```python
from build123d import *

# Parameters (mm, degrees)
F0_R      = 11
F1_DEPTH  = 7
F2_F1_R   = 2.54
F2_F2_R   = 2.54
F7_DEPTH  = 7.001
F8_DEPTH  = 7.001
F9_DEPTH  = 7.001
F10_DEPTH = 7.001


with BuildPart() as f1:
    # F0 (on Top) → F1 (new body)
    with BuildSketch(Plane.XY):
        Polygon((-46.5175881982, -16.4707175266), (1.3742837651, -16.4707175266), (47.8816837651, -16.4707175266), (38.1750466591, -6.3388262363), (28.4684095532, 3.7930650539), (38.1750466591, 13.9249563442), (47.8816837651, 24.0568476345), (1.3742837651, 24.0568476345), (-46.5175881982, 24.0568476345), (-36.8075984385, 13.9249563442), (-27.0976086789, 3.7930650539), (-36.8075984385, -6.3388262363), align=None)
        with Locations((1.3742837651, 3.7930650539)):
            Circle(F0_R, mode=Mode.SUBTRACT)
    extrude(amount=F1_DEPTH)

    # F2: fillet of radius 2.54 on 10 edges, made by hand

    # F2_f1
    f2_f1_edges = [f1.edges().sort_by_distance(p)[0] for p in [
        (28.4684095532, 3.7930650539, 3.5),
        (-27.0976086789, 3.7930650539, 3.5),
    ]]
    fillet(f2_f1_edges, radius=F2_F1_R)

    # F2_f2
    f2_f2_edges = [f1.edges().sort_by_distance(p)[0] for p in [
        (0.6820477835, -16.4707175266, 7),
        (0.6820477835, 24.0568476345, 7),
        (0.6820477835, 24.0568476345, 0),
        (0.6820477835, -16.4707175266, 0),
        (39.0167452033, -7.2174001498, 7),
        (-37.649739308, 14.8036884491, 7),
        (-37.649739308, -7.2175583413, 0),
        (39.0167452033, 14.8035302576, 0),
        (29.4459362755, 3.7930650539, 0),
        (-28.0757168957, 3.7930650539, 0),
        (-28.0757168957, 3.7930650539, 7),
        (29.4459362755, 3.7930650539, 7),
    ]]
    fillet(f2_f2_edges, radius=F2_F2_R)

    # F3 (on face) → F7 (cut, through all)
    with BuildSketch(Plane.XY.offset(7)):
        Polygon((-12.7487120452, 8.4079941735), (-12.7487120452, 16.6059941735), (-19.8483883054, 20.7049941735), (-26.9480645657, 16.6059941735), (-26.9480645657, 8.4079941735), (-19.8483883054, 4.3089941735), align=None)
    extrude(amount=-F7_DEPTH, mode=Mode.SUBTRACT)

    # F4 (on face) → F8 (cut, through all)
    with BuildSketch(Plane.XY.offset(7)):
        Polygon((-12.8069793108, -8.9152967557), (-12.8069793108, -0.7172967557), (-19.906655571, 3.3817032443), (-27.0063318312, -0.7172967557), (-27.0063318312, -8.9152967557), (-19.906655571, -13.0142967557), align=None)
    extrude(amount=-F8_DEPTH, mode=Mode.SUBTRACT)

    # F6 (on face) → F9 (cut, through all)
    with BuildSketch(Plane.XY.offset(7)):
        Polygon((27.5151642737, -8.7466302544), (27.5151642737, -0.5486302544), (20.4154880135, 3.5503697456), (13.3158117533, -0.5486302544), (13.3158117533, -8.7466302544), (20.4154880135, -12.8456302544), align=None)
    extrude(amount=-F9_DEPTH, mode=Mode.SUBTRACT)

    # F5 (on face) → F10 (cut, through all)
    with BuildSketch(Plane.XY.offset(7)):
        Polygon((27.5004574447, 8.5391272614), (27.5004574447, 16.7371272614), (20.4007811844, 20.8361272614), (13.3011049242, 16.7371272614), (13.3011049242, 8.5391272614), (20.4007811844, 4.4401272614), align=None)
    extrude(amount=-F10_DEPTH, mode=Mode.SUBTRACT)


solid = f1.part
```
Check sheet for the modelled part. Datum: model origin and axes. Units: mm. A direction names the side the tool comes from. Round coordinates to 2 decimals unless told otherwise and drop trailing zeros. Order: outer loops, then holes, each group sorted by start corner. A loop starts at its lowest first (then second) coordinate and runs counter-clockwise, first axis right, second up. Notation, with made-up numbers: (23, 45.5) -> (28, 45.5) arc R13 cw to (28, 68.5) -> close; hole circle Ø8 at (16.25, 34). An arc over 180 degrees is marked (long way). One line per item, written item: value. Start each with the question number.
Q1. Cross-section at B-B (x = 9). Record the boundary of the cut face in (y, z), and give its area (3 significant figures).
Q2. Cross-section at A-A (x = 25.5). Record the boundary of the cut face in (y, z), and give its area (3 significant figures).
Q3. Cross-section at C-C (y = -11.5). Give the number of separate pieces and of enclosed holes in the cut face, and give its area (3 significant figures).
Q4. Set-up check for faces 1 (the face through (-23.41, 1.36, 3.55)), 2 (the face through (29.446, 3.766, 3.513)), 3 (the face through (38.34, -7.62, 0.72)), 4 (the face through (-37.53, -7.09, 3.49)), 5 (the face through (-37.25, -7.85, 0.76)): record each of +Z, -Z, +X, -X, +Y, -Y from which the full face is reachable in a straight line by a thin tool's end or side.
Q5. Mould release check, pull along Y, two halves, no side actions. Record for faces 6 (the face through (-9, 8, 0)), 7 (the face through (1, 24.057, 3)), 8 (the face through (1.343, -15.707, 0.724)), 9 (the face through (23.9, 6.46, 3.55)): pulls with the +Y half, pulls with the -Y half, needs draft (parallel to the pull), parting line crosses it, or undercut.
Q6. Gauge pin test, flat ends, axial feed: pin 1 Ø2 at (y, z) = (12, 2) entering from +X; pin 2 Ø3.5 at (y, z) = (-6, 2.5) entering from -X; pin 3 Ø2 at (y, z) = (11, 4) entering from -X. Record the tip position at first contact, or that the pin passes through.
Q7. Thickness scan on line 1 (Y direction, x = -26, z = 1.25); line 2 (Y direction, x = -15, z = 1); line 3 (X direction, y = -5, z = 2.75). Record the ranges inside material, lowest first.
Completed:
1. outline: (-16.47, 2.54) arc R2.54 ccw to (-13.93, 0) -> (-4.13, 0) -> (-4.13, 7) -> (-13.93, 7) arc R2.54 ccw to (-16.47, 4.46) -> close; (11.72, 0) -> (21.52, 0) arc R2.54 ccw to (24.06, 2.54) -> (24.06, 4.46) arc R2.54 ccw to (21.52, 7) -> (11.72, 7) -> close
1. area: 167 mm²
2. outline: (-16.47, 2.54) arc R2.54 ccw to (-13.93, 0) -> (-9.91, 0) -> (-9.91, 7) -> (-13.93, 7) arc R2.54 ccw to (-16.47, 4.46) -> close; (0.61, 0) -> (7.38, 0) -> (7.38, 7) -> (0.61, 7) -> close; (17.89, 0) -> (21.52, 0) arc R2.54 ccw to (24.06, 2.54) -> (24.06, 4.46) arc R2.54 ccw to (21.52, 7) -> (17.89, 7) -> close
2. area: 131 mm²
3. separate pieces: 3
3. enclosed holes: 0
3. area: 517 mm²
4. face 1: +Z, -Z
4. face 2: +Z, -Z, +X
4. face 3: -Z, +X
4. face 4: +Z, -Z, -X
4. face 5: -Z, -X
5. face 6: needs draft
5. face 7: pulls with the +Y half
5. face 8: pulls with the -Y half
5. face 9: undercut
6. pin 1: stops at x = 37.24
6. pin 2: stops at x = -38.16
6. pin 3: stops at x = -34.96
7. line 1: y = -16.12 to -9.5, -0.14 to 7.86, 17.15 to 23.7
7. line 2: y = -15.95 to -10.18, 0.55 to 7.11, 17.91 to 23.54
7. line 3: x = -35.52 to -27.01, -12.81 to -5.23, 7.98 to 13.32, 27.52 to 36.89
